Check sheet for the modelled part. Datum: model origin and axes. Units: mm. Face numbers are marked on the shaded views. A direction names the side the tool comes from. Round coordinates to 2 decimals unless told otherwise and drop trailing zeros. Write each loop counter-clockwise with the first axis right and the second up, starting at its lowest first coordinate (ties: lowest second). Pieces come first, ordered by that corner, then holes. Notation, with made-up numbers: (63, 51.25) -> (98, 51.25) arc R19 ccw to (98, 87.25) -> close; hole circle Ø3 at (50.5, -39.5). An arc over 180 degrees is marked (long way). One line per item, written item: value. Start each with the question number.
```python
from build123d import *

# Parameters (mm, degrees)
TAGLIO_ESTRUSIONE1_DEPTH = 1.5


with BuildPart() as part:
    # Schizzo1 → Rivoluzione1 (revolve)
    with BuildSketch(Plane.XY, mode=Mode.PRIVATE) as rivoluzione1_sk:
        with BuildLine():
            Line((0, 0), (1.24, 0))
            Line((1.24, 0), (1.24, 4.46))
            Line((1.24, 4.46), (2.25, 4.46))
            Line((2.25, 4.46), (2.25, 5.46))
            Line((2.25, 5.46), (1.3, 6.008482756))
            Line((1.3, 6.008482756), (1.3, 8.008482756))
            ThreePointArc((1.3, 8.008482756), (1.854378023, 10.195968379), (0, 11.481935132))
            Line((0, 11.481935132), (0, 0))
        make_face()
    revolve(rivoluzione1_sk.sketch.rotate(Axis((0, 0, 0), (0, 1, 0)), 90), axis=Axis((0, 0, 0), (0, 1, 0)))

    # TaglioSuperficie1
    split(bisect_by=Plane(origin=(0, 11.1, 0), x_dir=(-1, 0, 0), z_dir=(0, -1, 0)), keep=Keep.TOP)

    # Schizzo2 → Taglio-Estrusione1 (cut)
    with BuildSketch(Plane(origin=(0, 11.1, 0), x_dir=(-1, 0, 0), z_dir=(0, -1, 0))):
        Polygon((-0.416334141, -0.759385201), (0.449479805, -0.740248543), (0.865813946, 0.019136658), (0.416334141, 0.759385201), (-0.449479805, 0.740248543), (-0.865813946, -0.019136658), align=None)
    extrude(amount=TAGLIO_ESTRUSIONE1_DEPTH, mode=Mode.SUBTRACT)


solid = part.part
```
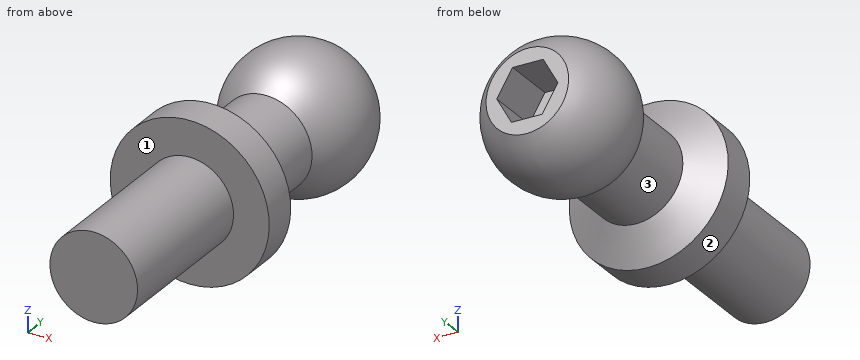
1. Material ranges on probe 1 along Y at (x, z) = (0.3, -0.05); probe 2 along Y at (x, z) = (1.25, -1.4); probe 3 along Y at (x, z) = (1.1, -0.8), recorded low to high.
2. Depth check by flat-ended pin: pin 1 Ø1 at (x, z) = (0.5, 0.5) entering from -Y; pin 2 Ø1.5 at (x, y) = (1.5, 2.5) entering from +Z. Enter the tip coordinate at first touch or a pass-through.
3. Cross-section at B-B (y = 7.5). Record the cut outline in (x, z).
4. Cross-section at A-A (x = 0). Record the cut outline in (y, z).
5. Access from +Z, -Z, +X, -X, +Y, -Y to the whole of each face (thin tool, end or side, straight path). Record for the marked faces 1, 2 and 3.
6. Cross-section at C-C (y = 5.75). Record the cut outline in (x, z), plus the area to 3 significant figures.
Working result:
1. probe 1: y = 0 to 9.6
1. probe 2: y = 4.46 to 5.68, 8.87 to 10.13
1. probe 3: y = 4.46 to 5.97, 8.06 to 10.94
2. pin 1: stops at y = 0
2. pin 2: stops at z = 0.99
3. outline: circle Ø2.6 at (0, 0)
4. outline: (0, -1.24) -> (4.46, -1.24) -> (4.46, -2.25) -> (5.46, -2.25) -> (6.01, -1.3) -> (8.01, -1.3) arc R1.98 ccw to (11.1, -1.17) -> (11.1, -0.75) -> (9.6, -0.75) -> (9.6, 0.75) -> (11.1, 0.75) -> (11.1, 1.17) arc R1.98 ccw to (8.01, 1.3) -> (6.01, 1.3) -> (5.46, 2.25) -> (4.46, 2.25) -> (4.46, 1.24) -> (0, 1.24) -> close
5. face 1: -Y
5. face 2: +Y, -Y
5. face 3: none
6. outline: circle Ø3.5 at (0, 0)
6. area: 9.60 mm^2
